Part model, mm, in its own coordinate system. Round coordinates to 2 decimals unless told otherwise and drop trailing zeros. Loops run counter-clockwise (first coordinate to the right, second up) from the corner with the lowest first, then second, coordinate; pieces in that order, holes last. Notation, with made-up numbers: (63.25, -32) -> (70.25, -32) arc R23 ccw to (70.25, -7) -> close; hole circle Ø6 at (72, 59.5). An arc over 180 degrees is marked (long way). Use a Markdown table: item, result. Add a question column.
Item 1: Two-plate mould, pull along Z, no slides. Class faces 1 (the face through (-1, 0, -36)), 2 (the face through (-30, 2, -60)), 3 (the face through (0.143, 2.028, -78.247)): pulls with the +Z half, pulls with the -Z half, needs draft (parallel to the pull), parting line crosses it, or undercut.
Item 2: Probe line 1 (X direction, y = 1.35, z = -15); line 2 (Z direction, x = -1, y = 3.3); line 3 (X direction, y = 1.8, z = -75). List the from-to ranges inside material, lowest first. Write a range as [from, to].
Item 3: Cut at C-C, the plane y = 1.6. List the corners of the cut face in (x, z), plus the area to 3 significant figures.
Item 4: Cut at D-D, the plane z = -15. List the corners of the cut face in (x, y), plus the area to 3 significant figures.
Item 5: Cut at A-A, the plane z = -75. List the corners of the cut face in (x, y), plus the area to 3 significant figures.
Item 6: Flat gauge pins, fed straight in: pin 1 (4 mm diameter, centred on x = 0, z = -15, fed in from -Y); pin 2 (1 mm diameter, centred on y = 2, z = -58.5, fed in from -X). Where does each tip first touch, or does it go through?
Item 7: Cut at B-B, the plane x = 30. List the corners of the cut face in (y, z), plus the area to 3 significant figures.
```python
from build123d import *

# Parameters (mm, degrees)
BOSS_EXTRUDE1_DEPTH = 4
SKETCH2_R           = 3.25
CUT_EXTRUDE1_DEPTH  = 101.702532242


with BuildPart() as part:
    # Sketch1 → Boss-Extrude1 (new body)
    with BuildSketch(Plane(origin=(0, 0, 0), x_dir=(1, 0, 0), z_dir=(0, 1, 0))):
        Polygon((-45, 0), (45, 0), (45, 30), (15, 90), (-15, 90), (-45, 30), align=None)
    extrude(amount=BOSS_EXTRUDE1_DEPTH)

    # Sketch2 → Cut-Extrude1 (cut, through all)
    with BuildSketch(Plane(origin=(0, 4, 0), x_dir=(1, 0, 0), z_dir=(0, 1, 0))):
        with Locations(Location((0, 75, 0), (0, 0, 270))):
            Circle(SKETCH2_R)
        with Locations(Location((0, 45, 0), (0, 0, 270))):
            Circle(SKETCH2_R)
        with Locations(Location((0, 15, 0), (0, 0, 270))):
            Circle(SKETCH2_R)
        with Locations(Location((30, 15, 0), (0, 0, 270))):
            Circle(SKETCH2_R)
        with Locations(Location((-30, 15, 0), (0, 0, 270))):
            Circle(SKETCH2_R)
    extrude(amount=-CUT_EXTRUDE1_DEPTH, mode=Mode.SUBTRACT)


solid = part.part
```
A:
| question | item | result |
|---|---|---|
| 1 | face 1 | needs draft |
| 1 | face 2 | pulls with the -Z half |
| 1 | face 3 | undercut |
| 2 | line 1 | x = [-45, -33.25], [-26.75, -3.25], [3.25, 26.75], [33.25, 45] |
| 2 | line 2 | z = [-90, -78.09], [-71.91, -48.09], [-41.91, -18.09], [-11.91, 0] |
| 2 | line 3 | x = [-22.5, -3.25], [3.25, 22.5] |
| 3 | outline | (-45, -30) -> (-15, -90) -> (15, -90) -> (45, -30) -> (45, 0) -> (-45, 0) -> close; hole circle Ø6.5 at (-30, -15); hole circle Ø6.5 at (0, -75); hole circle Ø6.5 at (0, -45); hole circle Ø6.5 at (0, -15); hole circle Ø6.5 at (30, -15) |
| 3 | area | 6,130 mm^2 |
| 4 | outline | (-45, 0) -> (-33.25, 0) -> (-33.25, 4) -> (-45, 4) -> close; (-26.75, 0) -> (-3.25, 0) -> (-3.25, 4) -> (-26.75, 4) -> close; (3.25, 0) -> (26.75, 0) -> (26.75, 4) -> (3.25, 4) -> close; (33.25, 0) -> (45, 0) -> (45, 4) -> (33.25, 4) -> close |
| 4 | area | 282 mm^2 |
| 5 | outline | (-22.5, 0) -> (-3.25, 0) -> (-3.25, 4) -> (-22.5, 4) -> close; (3.25, 0) -> (22.5, 0) -> (22.5, 4) -> (3.25, 4) -> close |
| 5 | area | 154 mm^2 |
| 6 | pin 1 | passes through |
| 6 | pin 2 | stops at x = -31 |
| 7 | outline | (0, -60) -> (4, -60) -> (4, -18.25) -> (0, -18.25) -> close; (0, -11.75) -> (4, -11.75) -> (4, 0) -> (0, 0) -> close |
| 7 | area | 214 mm^2 |
